from build123d import *

# Parameters (mm, degrees)
SKETCH1_W           = 80
SKETCH1_H           = 50
SKETCH1_R           = 5.5
BOSS_EXTRUDE1_DEPTH = 5
SKETCH3_R           = 1.5
CUT_EXTRUDE1_DEPTH  = 5


with BuildPart() as part:
    # Sketch1 → Boss-Extrude1 (new body)
    with BuildSketch(Plane(origin=(0, 0, 0), x_dir=(1, 0, 0), z_dir=(0, 1, 0))):
        with Locations((40, 25)):
            Rectangle(SKETCH1_W, SKETCH1_H)
        with Locations(Location((45, 25, 0), (0, 0, 270))):
            Circle(SKETCH1_R, mode=Mode.SUBTRACT)
        with BuildLine():
            Line((10, 43), (20, 43))
            ThreePointArc((20, 43), (23, 40), (20, 37))
            Line((20, 37), (10, 37))
            ThreePointArc((10, 37), (7, 40), (10, 43))
        make_face(mode=Mode.SUBTRACT)
        with BuildLine():
            Line((10, 13), (20, 13))
            ThreePointArc((20, 13), (23, 10), (20, 7))
            Line((20, 7), (10, 7))
            ThreePointArc((10, 7), (7, 10), (10, 13))
        make_face(mode=Mode.SUBTRACT)
    extrude(amount=BOSS_EXTRUDE1_DEPTH)

    # Sketch3 → Cut-Extrude1 (cut)
    with BuildSketch(Plane.XZ):
        with Locations(Location((45, -17, 0), (0, 0, 270))):
            Circle(SKETCH3_R)
        with Locations(Location((53, -25, 0), (0, 0, 270))):
            Circle(SKETCH3_R)
        with Locations(Location((45, -33, 0), (0, 0, 270))):
            Circle(SKETCH3_R)
        with Locations(Location((37, -25, 0), (0, 0, 270))):
            Circle(SKETCH3_R)
    extrude(amount=-CUT_EXTRUDE1_DEPTH, mode=Mode.SUBTRACT)


solid = part.part
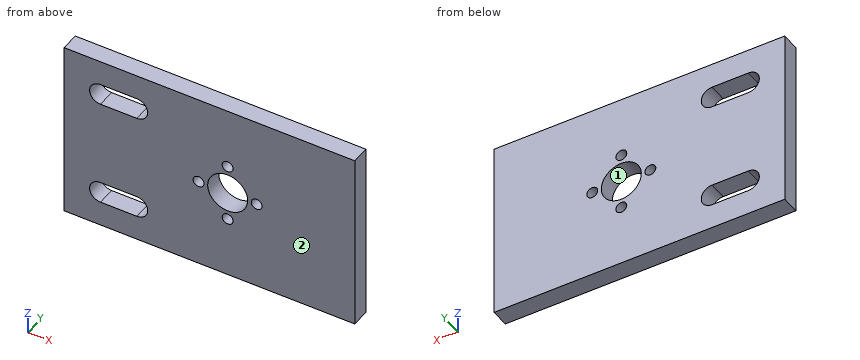
Input: part model. Units: mm. Frame: model coordinates. Face numbers are marked on the shaded views. Coordinates: 2 decimals unless noted, no trailing zeros. Loops run counter-clockwise (first coordinate to the right, second up) from the corner with the lowest first, then second, coordinate; pieces in that order, holes last.
Q1. Cut plane C-C (x = 53). Output: boundary loops of the cut face in (y, z), then the cut area to 3 significant figures.
Q2. Cut plane D-D (y = 2.1). Output: boundary loops of the cut face in (x, z), then the cut area to 3 significant figures.
Q3. Cut plane B-B (z = -10). Output: boundary loops of the cut face in (x, y).
Q4. Material intervals for line 1 (X direction, y = 1.85, z = -25); line 2 (X direction, y = 0.65, z = -10); line 3 (X direction, y = 3.55, z = -17), sorted ascending.
Q5. Draft query along Z for the marked faces 1 and 2. Return one class per face: +Z half, -Z half, draft (parallel to the pull), parting line (faces both ways), or undercut.
Q6. Cut plane A-A (x = 18.5). Output: boundary loops of the cut face in (y, z).
Working result:
1. outline: (0, -50) - (5, -50) - (5, -26.5) - (0, -26.5) - close; (0, -23.5) - (5, -23.5) - (5, 0) - (0, 0) - close
1. area: 235 mm2
2. outline: (0, -50) - (80, -50) - (80, 0) - (0, 0) - close; hole (10, -43) - (20, -43) arc R3 ccw to (20, -37) - (10, -37) arc R3 ccw to start; hole (10, -13) - (20, -13) arc R3 ccw to (20, -7) - (10, -7) arc R3 ccw to start; hole circle Ø3 at (37, -25); hole circle Ø11 at (45, -25); hole circle Ø3 at (45, -33); hole circle Ø3 at (45, -17); hole circle Ø3 at (53, -25)
2. area: 3,700 mm2
3. outline: (0, 0) - (7, 0) - (7, 5) - (0, 5) - close; (23, 0) - (80, 0) - (80, 5) - (23, 5) - close
4. line 1: x = 0 to 35.5, 38.5 to 39.5, 50.5 to 51.5, 54.5 to 80
4. line 2: x = 0 to 7, 23 to 80
4. line 3: x = 0 to 43.5, 46.5 to 80
5. face 1: undercut
5. face 2: draft
6. outline: (0, -50) - (5, -50) - (5, -43) - (0, -43) - close; (0, -37) - (5, -37) - (5, -13) - (0, -13) - close; (0, -7) - (5, -7) - (5, 0) - (0, 0) - close
